Geometry: final body of the model. Coordinates: model frame, mm. Face numbers are marked on the shaded views. A direction names the side the tool comes from. Coordinates: 2 decimals unless noted, no trailing zeros. Write each loop counter-clockwise with the first axis right and the second up, starting at its lowest first coordinate (ties: lowest second). Pieces come first, ordered by that corner, then holes. Notation, with made-up numbers: (11.25, 57) -> (18.25, 57) arc R22 ccw to (18.25, 87) -> close; hole circle Ø8 at (47, 17). An arc over 180 degrees is marked (long way). One line per item, written item: value.
```python
from build123d import *

# Parameters (mm, degrees)
SKETCH1_W           = 218
SKETCH1_H           = 30
BOSS_EXTRUDE1_DEPTH = 5
FILLET1_R           = 20
SKETCH4_R           = 5
CUT_EXTRUDE2_DEPTH  = 119.749210232
BOSS_EXTRUDE2_DEPTH = 20
CHAMFER2_SIZE       = 5
FILLET3_R           = 5


with BuildPart() as part:
    # Sketch1 → Boss-Extrude1 (new, symmetric)
    with BuildSketch(Plane.XY):
        Rectangle(SKETCH1_W, SKETCH1_H)
    extrude(amount=BOSS_EXTRUDE1_DEPTH, both=True)

    # Fillet1
    fillet1_edges = [part.edges().sort_by_distance(p)[0] for p in [
        (109, -15, 0),
        (-109, -15, 0),
    ]]
    fillet(fillet1_edges, radius=FILLET1_R)

    # Sketch3 → Revolve1 (revolve)
    with BuildSketch(Plane(origin=(-61.85, 0, 0), x_dir=(0, 0, -1), z_dir=(1, 0, 0)), mode=Mode.PRIVATE) as revolve1_sk:
        Polygon((-20.498711306, 18.495190528), (-24.248711306, 12), (10.392304845, -8), (14.142304845, -1.504809472), align=None)
    revolve(revolve1_sk.sketch.rotate(Axis((-61.85, 12, 24.248711306), (0, -0.49999999999999767, -0.86602540378444)), 180), axis=Axis((-61.85, 12, 24.248711306), (0, -0.49999999999999767, -0.86602540378444)))

    # Sketch4 → Cut-Extrude2 (cut, through all)
    with BuildSketch(Plane(origin=(0, 13.5, 23.382685902), x_dir=(1, 0, 0), z_dir=(0, 0.4999999999999978, 0.86602540378444))):
        with Locations(Location((-61.85, -1.732050808, 0), (0, 0, 270))):
            Circle(SKETCH4_R)
    extrude(amount=-CUT_EXTRUDE2_DEPTH, mode=Mode.SUBTRACT)

    # Sketch5 → Boss-Extrude2 (add, symmetric)
    with BuildSketch(Plane(origin=(0, 0, 0), x_dir=(0, 0, -1), z_dir=(1, 0, 0))):
        Polygon((5, -15), (-5, -15), (-33.867513459, -65), (-91.641016151, -65), (-91.641016151, -75), (-29.641016151, -75), align=None)
    extrude(amount=BOSS_EXTRUDE2_DEPTH, both=True)

    # Chamfer2
    chamfer2_edges = [part.edges().sort_by_distance(p)[0] for p in [
        (-109, 15, 0),
        (109, 15, 0),
    ]]
    chamfer(chamfer2_edges, length=CHAMFER2_SIZE)

    # Fillet3
    fillet3_edges = [part.edges().sort_by_distance(p)[0] for p in [
        (-109, 10, 0),
        (104, 15, 0),
        (-104, 15, 0),
        (109, 10, 0),
    ]]
    fillet(fillet3_edges, radius=FILLET3_R)


solid = part.part
```
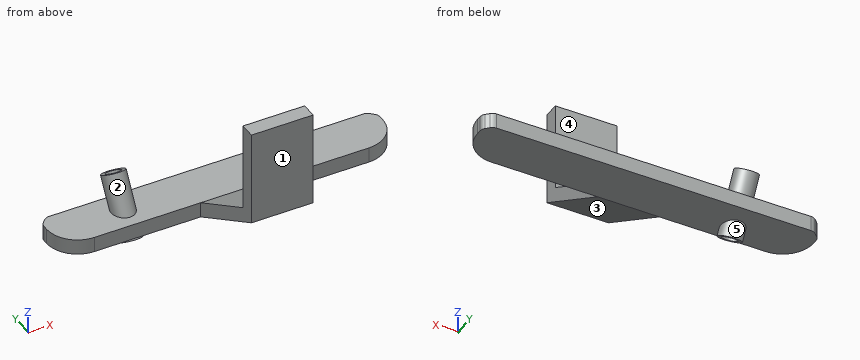
(1) Section A-A (z = 58). Return the cut outline in (x, y).
Responses:
outline: (-20, -75) -> (20, -75) -> (20, -65) -> (-20, -65) -> close
(2) Section B-B (x = 52.5). Return the cut outline in (y, z), then the cut area to 3 significant figures.
Responses:
outline: (-15, -5) -> (15, -5) -> (15, 5) -> (-15, 5) -> close
area: 300 mm2
(3) First-contact query: pin 1 (12 mm diameter, centred on y = 8.5, z = 27, fed in from +X); pin 2 (3 mm diameter, centred on x = -19, z = -1, fed in from +Y); pin 3 (8 mm diameter, centred on x = 41, z = 2, fed in from -Y); pin 4 (5 mm diameter, centred on x = 55.5, y = -18.5, fed in from +Z). Flat tips, straight axial feed; report the tip coordinate or a pass-through.
Responses:
pin 1: stops at x = -54.35
pin 2: stops at y = 15
pin 3: stops at y = -15
pin 4: passes through
(4) Section C-C (z = 18). State how many separate pieces and enclosed holes the cut face has, then the cut area to 3 significant figures.
Responses:
separate pieces: 2
enclosed holes: 1
area: 806 mm2
(5) Line query: line 1 (Z direction, x = -97, y = -7); line 2 (X direction, y = -30, z = 5.5); line 3 (X direction, y = 11.5, z = 4). Output: solid intervals per line, ascending. Write a range as [from, to].
Responses:
line 1: z = [-5, 5]
line 2: x = [-20, 20]
line 3: x = [-107.5, 107.5]
(6) Reachability of the marked faces 4 and 5 from +Z, -Z, +X, -X, +Y, -Y: full face, straight path, thin tool, end or side. Return the list, or none.
Responses:
face 4: +Z, +X, -X, +Y
face 5: none
(7) Pull-direction query (Z, two-part tool) for the marked faces 1, 2 and 3; classes: released by +Z, released by -Z, zero draft, split by the parting line, or undercut.
Responses:
face 1: zero draft
face 2: undercut
face 3: released by -Z
